```python
from build123d import *

# Parameters (mm, degrees)
SKETCH2_W           = 17
SKETCH2_H           = 2.75
BOSS_EXTRUDE1_DEPTH = 8
BOSS_EXTRUDE3_DEPTH = 8
SKETCH5_R           = 3
CUT_EXTRUDE1_DEPTH  = 3
SKETCH6_R           = 1.65
CUT_EXTRUDE2_DEPTH  = 8
FILLET14_R          = 2
FILLET15_R          = 2
FILLET16_R          = 2
SKETCH7_W           = 18
SKETCH7_H           = 10
CUT_EXTRUDE3_DEPTH  = 1
FILLET18_R          = 1.4
BOSS_EXTRUDE4_DEPTH = 10
SKETCH10_R          = 4.25
CUT_EXTRUDE4_DEPTH  = 8
FILLET17_R          = 2
FILLET19_R          = 5
SKETCH11_W          = 35
SKETCH11_H          = 13.55262527
CUT_EXTRUDE5_DEPTH  = 46.43556564


with BuildPart() as part:
    # Sketch2 → Boss-Extrude1 (new body)
    with BuildSketch(Plane(origin=(0, 0, 0), x_dir=(1, 0, 0), z_dir=(0, 1, 0))):
        Rectangle(SKETCH2_W, SKETCH2_H)
    extrude(amount=BOSS_EXTRUDE1_DEPTH)

    # Sketch3 → Boss-Extrude3 (add)
    with BuildSketch(Plane(origin=(0, 0, 0), x_dir=(1, 0, 0), z_dir=(0, 1, 0))):
        Polygon((4, -9.375), (17.5, -9.375), (17.5, -24.375), (-17.5, -24.375), (-17.5, -9.375), (-4, -9.375), (-4, -1.375), (4, -1.375), align=None)
    extrude(amount=BOSS_EXTRUDE3_DEPTH)

    # Sketch5 → Cut-Extrude1 (cut)
    with BuildSketch(Plane.XZ):
        with Locations(Location((13, 19.375, 0), (0, 0, 270))):
            Circle(SKETCH5_R)
        with Locations(Location((-13, 19.375, 0), (0, 0, 270))):
            Circle(SKETCH5_R)
    extrude(amount=-CUT_EXTRUDE1_DEPTH, mode=Mode.SUBTRACT)

    # Sketch6 → Cut-Extrude2 (cut)
    with BuildSketch(Plane.XZ):
        with Locations(Location((-13, 19.375, 0), (0, 0, 270))):
            Circle(SKETCH6_R)
        with Locations(Location((13, 19.375, 0), (0, 0, 270))):
            Circle(SKETCH6_R)
    extrude(amount=-CUT_EXTRUDE2_DEPTH, mode=Mode.SUBTRACT)

    # Fillet14
    fillet14_edges = [part.edges().sort_by_distance(p)[0] for p in [
        (-4, 4, 9.375),
    ]]
    fillet(fillet14_edges, radius=FILLET14_R)

    # Fillet15
    fillet15_edges = [part.edges().sort_by_distance(p)[0] for p in [
        (4, 4, 9.375),
    ]]
    fillet(fillet15_edges, radius=FILLET15_R)

    # Fillet16
    fillet16_edges = [part.edges().sort_by_distance(p)[0] for p in [
        (-4, 4, 1.375),
    ]]
    fillet(fillet16_edges, radius=FILLET16_R)

    # Sketch7 → Cut-Extrude3 (cut)
    with BuildSketch(Plane(origin=(0, 8, 0), x_dir=(1, 0, 0), z_dir=(0, 1, 0))):
        with Locations((0, -19.375)):
            Rectangle(SKETCH7_W, SKETCH7_H)
    extrude(amount=-CUT_EXTRUDE3_DEPTH, mode=Mode.SUBTRACT)

    # Fillet18
    fillet18_edges = [part.edges().sort_by_distance(p)[0] for p in [
        (8.5, 8, 0),
        (-8.5, 8, 0),
        (8.5, 0, 0),
        (-8.5, 0, 0),
    ]]
    fillet(fillet18_edges, radius=FILLET18_R)

    # Sketch9 → Boss-Extrude4 (add)
    with BuildSketch(Plane.XY.offset(24.375)):
        with BuildLine():
            Line((-17.5, 0), (-37.5, 0))
            Line((-37.5, 0), (-37.5, 6))
            ThreePointArc((-37.5, 6), (-31.5, 12), (-25.5, 6))
            Line((-25.5, 6), (-25.5, 5))
            Line((-25.5, 5), (-17.5, 5))
            Line((-17.5, 5), (-17.5, 0))
        make_face()
        with BuildLine():
            Line((25.5, 6), (25.5, 5))
            Line((25.5, 5), (17.5, 5))
            Line((17.5, 5), (17.5, 0))
            Line((17.5, 0), (37.5, 0))
            Line((37.5, 0), (37.5, 6))
            ThreePointArc((37.5, 6), (31.5, 12), (25.5, 6))
        make_face()
    extrude(amount=-BOSS_EXTRUDE4_DEPTH)

    # Sketch10 → Cut-Extrude4 (cut)
    with BuildSketch(Plane.XY.offset(24.375)):
        with Locations((-31.5, 6)):
            Circle(SKETCH10_R)
        with Locations(Location((31.5, 6, 0), (0, 0, 180))):
            Circle(SKETCH10_R)
    extrude(amount=-CUT_EXTRUDE4_DEPTH, mode=Mode.SUBTRACT)

    # Fillet17
    fillet17_edges = [part.edges().sort_by_distance(p)[0] for p in [
        (4, 4, 1.375),
    ]]
    fillet(fillet17_edges, radius=FILLET17_R)

    # Fillet19
    fillet19_edges = [part.edges().sort_by_distance(p)[0] for p in [
        (-37.5, 0, 19.375),
        (37.5, 0, 19.375),
    ]]
    fillet(fillet19_edges, radius=FILLET19_R)

    # Sketch11 → Cut-Extrude5 (cut, through all)
    with BuildSketch(Plane(origin=(0, 8, 0), x_dir=(1, 0, 0), z_dir=(0, 1, 0))):
        with Locations((0, -2.598687365)):
            Rectangle(SKETCH11_W, SKETCH11_H)
    extrude(amount=-CUT_EXTRUDE5_DEPTH, mode=Mode.SUBTRACT)


solid = part.part
```
Check sheet for the modelled part. Datum: model origin and axes. Units: mm. A direction names the side the tool comes from. Round coordinates to 2 decimals unless told otherwise and drop trailing zeros. Loops run counter-clockwise (first coordinate to the right, second up) from the corner with the lowest first, then second, coordinate; pieces in that order, holes last. Notation, with made-up numbers: (74.5, 5) - (117.5, 5) arc R26 cw to (117.5, 21) - close; hole circle Ø2 at (24.25, 89.25). An arc over 180 degrees is marked (long way). Answer as a JSON object with one key per item and string values. Group by question number.
Q1. Sectioned sample at A-A, the plane x = 13. Enter the section's corners in (y, z) (3 decimals), plus the area to 3 significant figures.
Q2. Sectioned sample at C-C, the plane x = 3. Enter the section's corners in (y, z) (3 decimals), plus the area to 3 significant figures.
Q3. Gauge pin test, flat ends, axial feed: P1, Ø1.8, axis at x = 14, z = 19, coming from the -Y side; P2, Ø2.5, axis at x = 13, z = 19.375, coming from the +Y side; P3, Ø8, axis at x = -13, z = 19.375, coming from the +Y side. Record the tip position at first contact, or that the pin passes through.
Q4. Set-up check for faces 4 (the face through (-17.5, 6, 15)), 5 (the face through (11.7, 3, 18.1)), 6 (the face through (22, 5, 19)), 7 (the face through (0, 4, 9.375)), 8 (the face through (-35.746, 6.187, 20.431)): record each of +Z, -Z, +X, -X, +Y, -Y from which the full face is reachable in a straight line by a thin tool's end or side.
Q5. Mould release check, pull along X, two halves, no side actions. Record for faces 1 (the face through (0, 0, 17)), 2 (the face through (35.746, 5.813, 20.431)), 3 (the face through (-36, 1.43, 19.3)): released by +X, released by -X, zero draft, split by the parting line, or undercut.
Q6. Sectioned sample at D-D, the plane x = 22.5. Enter the section's corners in (y, z) (3 decimals).
Q7. Sectioned sample at B-B, the plane x = -31.5. Enter the section's corners in (y, z) (3 decimals), plus the area to 3 significant figures.
Q8. Scan lines: line 1 along Y through (x, z) = (-31.5, 22.5); line 2 along X through (y, z) = (4, 17.5); line 3 along X through (y, z) = (6.5, 15.25). Record each from-to range of solid material in increasing order. Write a range as [from, to].
Solution:
{
 "1": {"outline": "(0, 9.375) - (8, 9.375) - (8, 17.725) - (3, 17.725) - (3, 16.375) - (0, 16.375) - close; (0, 22.375) - (3, 22.375) - (3, 21.025) - (8, 21.025) - (8, 24.375) - (0, 24.375) - close", "area": "85.5 mm²"},
 "2": {"outline": "(0, 9.375) - (8, 9.375) - (8, 14.375) - (7, 14.375) - (7, 24.375) - (0, 24.375) - close", "area": "110 mm²"},
 "3": {"P1": "stops at y = 3", "P2": "passes through", "P3": "stops at y = 8"},
 "4": {"face 4": "-Z, +Y", "face 5": "-Y", "face 6": "+Z, -Z, +Y", "face 7": "-Z, +X, -X, +Y, -Y", "face 8": "+Z"},
 "5": {"face 1": "zero draft", "face 2": "undercut", "face 3": "released by -X"},
 "6": {"outline": "(0, 14.375) - (5, 14.375) - (5, 24.375) - (0, 24.375) - close"},
 "7": {"outline": "(0, 14.375) - (12, 14.375) - (12, 24.375) - (10.25, 24.375) - (10.25, 16.375) - (1.75, 16.375) - (1.75, 24.375) - (0, 24.375) - close", "area": "52.0 mm²"},
 "8": {"line 1": "y = [0, 1.75], [10.25, 12]", "line 2": "x = [-37.4, -35.25], [-27.75, 27.75], [35.25, 37.4]", "line 3": "x = [-37.48, -25.52], [-17.5, 17.5], [25.52, 37.48]"}
}
